Verification items for the finished model (mm, model axes). A direction names the side the tool comes from. Give positions to 0.01 mm unless a question says otherwise; leave off trailing zeros. Loops run counter-clockwise (first coordinate to the right, second up) from the corner with the lowest first, then second, coordinate; pieces in that order, holes last. Notation, with made-up numbers: (12, 27.5) -> (41, 27.5) arc R28 ccw to (41, 55.5) -> close; hole circle Ø9 at (82, 25.25). An arc over 180 degrees is marked (long way). Answer in a Markdown table with one row per item. Add a question column.
Q1. Section check B-B on y = -6.25. Enter the section's corners in (x, z), and give its area (3 significant figures).
Q2. Set-up check for faces 1 (the face through (-25, -9, 112)), 2 (the face through (-50, -9, 127)), 3 (the face through (175, -10, 30)): record each of +Z, -Z, +X, -X, +Y, -Y from which the full face is reachable in a straight line by a thin tool's end or side.
Q3. Section check C-C on z = 109. Enter the section's corners in (x, y), and give its area (3 significant figures).
Q4. Section check A-A on x = 153.5. Enter the section's corners in (y, z).
Q5. Material ranges on probe 1 along Z at (x, y) = (75, -6); probe 2 along X at (y, z) = (-12.5, 126); probe 3 along Z at (x, y) = (173.5, -18), recorded low to high.
Q6. Gauge pin test, flat ends, axial feed: P1, Ø5, axis at y = -2.5, z = 93.5, coming from the -X side; P2, Ø3, axis at y = -5.5, z = 87.5, coming from the +X side; P3, Ø0.8, axis at x = 75, y = -9.5, coming from the -Z side. Record the tip position at first contact, or that the pin passes through.
Q7. Release check for a two-part mould opening along Z. For faces 4 (the face through (0, -9, 70)), 5 (the face through (73, -10, 0)), 6 (the face through (-50, -9, 15)), 7 (the face through (150, -9, 70)) record: pulls with the +Z half, pulls with the -Z half, needs draft (parallel to the pull), parting line crosses it, or undercut.
```python
from build123d import *

# Parameters (mm, degrees)
F0_W     = 150
F0_H     = 142
F0_R     = 0.5
F1_DEPTH = 19
F2_R     = 0.5
F3_DEPTH = 1
F4_R     = 0.5
F5_DEPTH = 1
F6_W     = 19
F6_H     = 30
F7_DEPTH = 50
F8_W     = 19
F8_H     = 30
F9_DEPTH = 50


with BuildPart() as f1:
    # F0 (on Front) → F1 (new body)
    with BuildSketch(Plane.XZ):
        with Locations((75, 71)):
            Rectangle(F0_W, F0_H)
        with Locations((75, 16)):
            Circle(F0_R, mode=Mode.SUBTRACT)
        with Locations((75, 126)):
            Circle(F0_R, mode=Mode.SUBTRACT)
    extrude(amount=F1_DEPTH)

    # F2 (on face) → F3 (cut)
    with BuildSketch(Plane(origin=(0, 0, 0), x_dir=(1, 0, 0), z_dir=(0, 0, -1))):
        with Locations((75, 9.5)):
            Circle(F2_R)
    extrude(amount=-F3_DEPTH, mode=Mode.SUBTRACT)

    # F4 (on face) → F5 (cut)
    with BuildSketch(Plane.XY.offset(142)):
        with Locations((75, -9.5)):
            Circle(F4_R)
    extrude(amount=-F5_DEPTH, mode=Mode.SUBTRACT)

    # F6 (on face) → F7 (join)
    with BuildSketch(Plane(origin=(0, 0, 0), x_dir=(0, -1, 0), z_dir=(-1, 0, 0))):
        with Locations((9.5, 127)):
            Rectangle(F6_W, F6_H)
        with Locations((9.5, 15)):
            Rectangle(F6_W, F6_H)
    extrude(amount=F7_DEPTH)

    # F8 (on face) → F9 (join)
    with BuildSketch(Plane.YZ.offset(150)):
        with Locations((-9.5, 15)):
            Rectangle(F8_W, F8_H)
        with Locations((-9.5, 127)):
            Rectangle(F8_W, F8_H)
    extrude(amount=F9_DEPTH)


solid = f1.part
```
Taken from the geometry:
| question | item | result |
|---|---|---|
| 1 | outline | (-50, 0) -> (200, 0) -> (200, 30) -> (150, 30) -> (150, 112) -> (200, 112) -> (200, 142) -> (-50, 142) -> (-50, 112) -> (0, 112) -> (0, 30) -> (-50, 30) -> close; hole circle Ø1 at (75, 16); hole circle Ø1 at (75, 126) |
| 1 | area | 27,300 mm² |
| 2 | face 1 | -X, +Y, -Y |
| 2 | face 2 | +Z, -Z, -X, +Y, -Y |
| 2 | face 3 | +X, +Y, -Y |
| 3 | outline | (0, -19) -> (150, -19) -> (150, 0) -> (0, 0) -> close |
| 3 | area | 2,850 mm² |
| 4 | outline | (-19, 0) -> (0, 0) -> (0, 30) -> (-19, 30) -> close; (-19, 112) -> (0, 112) -> (0, 142) -> (-19, 142) -> close |
| 5 | probe 1 | z = 0 to 15.5, 16.5 to 125.5, 126.5 to 142 |
| 5 | probe 2 | x = -50 to 74.5, 75.5 to 200 |
| 5 | probe 3 | z = 0 to 30, 112 to 142 |
| 6 | P1 | stops at x = 0 |
| 6 | P2 | stops at x = 150 |
| 6 | P3 | stops at z = 1 |
| 7 | face 4 | undercut |
| 7 | face 5 | pulls with the -Z half |
| 7 | face 6 | needs draft |
| 7 | face 7 | undercut |
